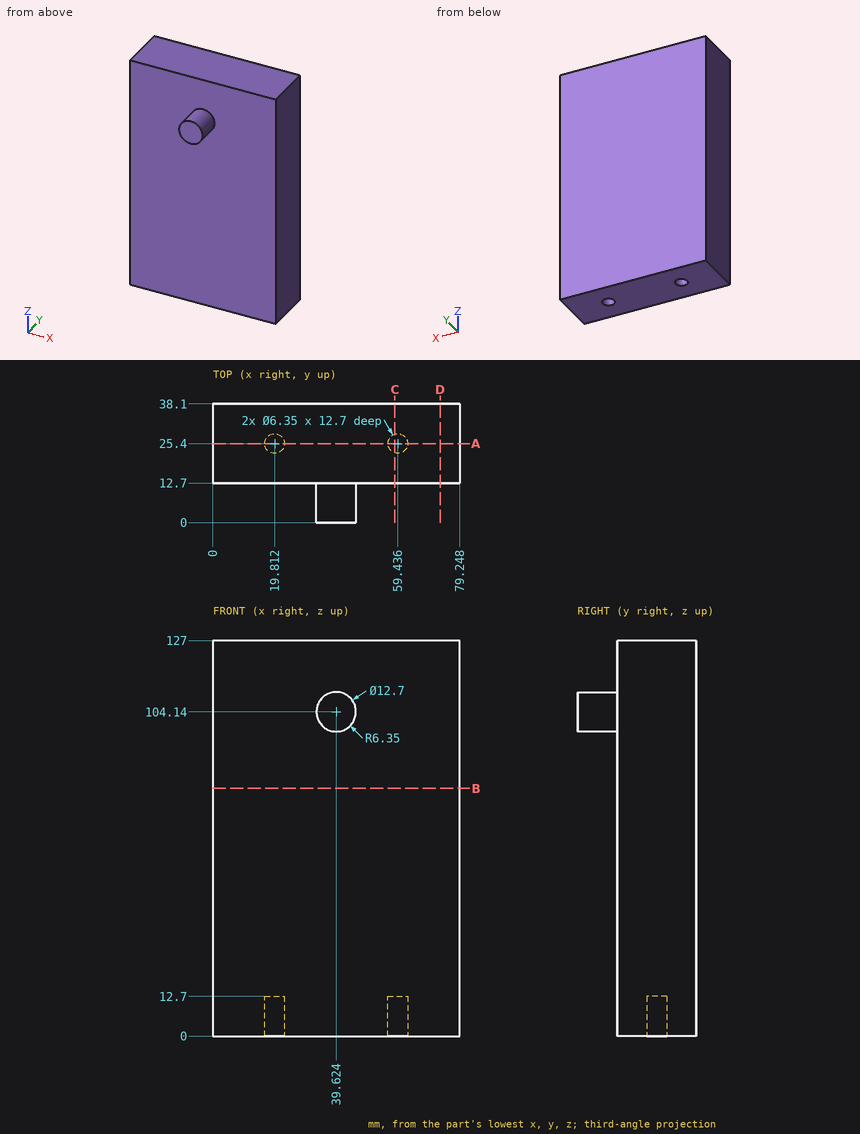
The drawing under review shows one solid part. Ordinate dimensions are in mm from its lowest x, y, z. Give positions to 0.01 mm unless a question says otherwise; leave off trailing zeros. Write each loop counter-clockwise with the first axis right and the second up, starting at its lowest first coordinate (ties: lowest second). Pieces come first, ordered by that corner, then holes. Notation, with made-up numbers: (13.25, 42) -> (37.25, 42) arc R15 cw to (37.25, 46) -> close; hole circle Ø6 at (89, -6.75). An arc over 180 degrees is marked (long way). Answer in a Markdown table with one row per item.
(1) Consider section B-B (z = 79.5). State the section outline as (x, y) points.
Results:
| item | result |
|---|---|
| outline | (0, 12.7) -> (79.25, 12.7) -> (79.25, 38.1) -> (0, 38.1) -> close |
(2) Clearance check with flat-ended pins moving along their axes: pin 1 (3 mm diameter, centred on x = 59, y = 25.5, fed in from -Z); pin 2 (3 mm diameter, centred on x = 58.5, z = 90.5, fed in from -Y). State where each tip first meets the part, or that it passes through.
Results:
| item | result |
|---|---|
| pin 1 | z = 12.7 |
| pin 2 | y = 12.7 |
(3) Consider section A-A (y = 25.4). State the section outline as (x, z) points.
Results:
| item | result |
|---|---|
| outline | (0, 0) -> (16.64, 0) -> (16.64, 12.7) -> (22.99, 12.7) -> (22.99, 0) -> (56.26, 0) -> (56.26, 12.7) -> (62.61, 12.7) -> (62.61, 0) -> (79.25, 0) -> (79.25, 127) -> (0, 127) -> close |
(4) To check wall thickness, follow probe 1 along X at (y, z) = (25, 4); probe 2 along Y at (x, z) = (26, 30); probe 3 along Z at (x, y) = (57, 26). State the ranges of each line that lie inside material, in increasing order.
Results:
| item | result |
|---|---|
| probe 1 | 0 to 16.66, 22.96 to 56.29, 62.59 to 79.25 |
| probe 2 | 12.7 to 38.1 |
| probe 3 | 12.7 to 127 |
(5) Consider section D-D (x = 73). State the section outline as (y, z) points.
Results:
| item | result |
|---|---|
| outline | (12.7, 0) -> (38.1, 0) -> (38.1, 127) -> (12.7, 127) -> close |
(6) Consider section C-C (x = 58.5). State the section outline as (y, z) points, then the cut area to 3 significant figures.
Results:
| item | result |
|---|---|
| outline | (12.7, 0) -> (22.37, 0) -> (22.37, 12.7) -> (28.43, 12.7) -> (28.43, 0) -> (38.1, 0) -> (38.1, 127) -> (12.7, 127) -> close |
| area | 3,150 mm2 |
